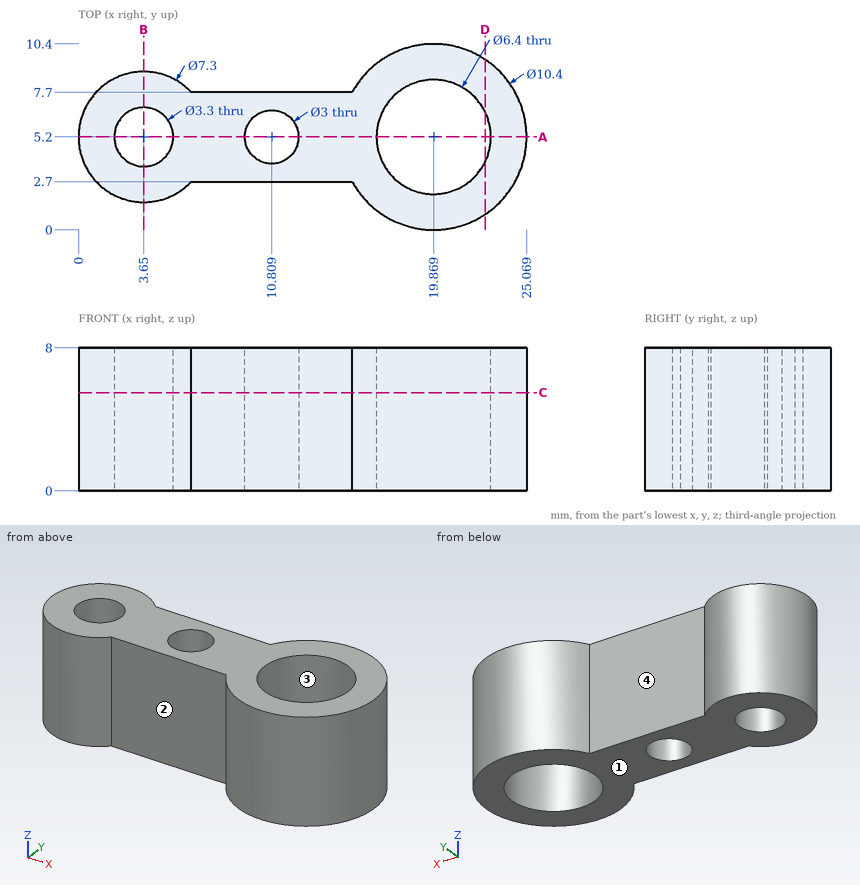
Could you check a few things on this drawing? It's one solid part, dimensions in mm from its lowest x, y, z. A direction names the side the tool comes from. Coordinates: 2 decimals unless noted, no trailing zeros. Order: outer loops, then holes, each group sorted by start corner. A loop starts at its lowest first (then second) coordinate and runs counter-clockwise, first axis right, second up. Notation, with made-up numbers: M 11,-26 L 51,-26 A24 ccw 51,-1 Z; hole C 10,-31.5 d1. An arc over 180 degrees is marked long. Use a Markdown table: item, result. Add a question column.
Q1. I want a section at D-D on x = 22.75. List the corners of the cut face in (y, z) for me.
Q2. I want a section at C-C on z = 5.5. List the corners of the cut face in (x, y) for me.
Q3. We'd pull the mould along X, two halves only. Please class the marked faces 1 and 2: pulls with the +X half, pulls with the -X half, needs draft (parallel to the pull), parting line crosses it, or undercut.
Q4. Which directions (+Z, -Z, +X, -X, +Y, -Y) give clear straight access to the entire face, cutting with the end or side of a thin tool? Please do the marked faces 3 and 4.
Q5. I'm going to push flat-ended pins straight in: pin 1 (2 mm diameter, centred on x = 18, z = 5, fed in from -Y); pin 2 (1.5 mm diameter, centred on x = 5, z = 7, fed in from -Y); pin 3 (4 mm diameter, centred on x = 14, y = 3, fed in from -Z); pin 4 (1 mm diameter, centred on x = 4.5, z = 3.5, fed in from +Y). Where does each tip first touch, or does it pass through?
Q6. I want a section at B-B on x = 3.65. List the corners of the cut face in (y, z) for me, then the cut area to 3 significant figures.
Q7. I want a section at A-A on y = 5.2. List the corners of the cut face in (x, z) for me.
Q8. If I drill on L1, parallel to X at y = 5.2, z = 6; L2, parallel to Y at x = 3.65, z = 3.5; L3, parallel to X at y = 4.5, z = 2 (1 decimal), over which ranges is the centre line in solid material (lowest first)?
Checked values:
| question | item | result |
|---|---|---|
| 1 | outline | M 0.87,0 L 3.81,0 L 3.81,8 L 0.87,8 Z; M 6.59,0 L 9.53,0 L 9.53,8 L 6.59,8 Z |
| 2 | outline | M 6.31,2.7 L 15.31,2.7 A5.2 ccw long 15.31,7.7 L 6.31,7.7 A3.65 ccw long Z; hole C 3.65,5.2 d3.3; hole C 10.81,5.2 d3; hole C 19.87,5.2 d6.4 |
| 3 | face 1 | needs draft |
| 3 | face 2 | undercut |
| 4 | face 3 | +Z, -Z |
| 4 | face 4 | +Z, -Z, +Y |
| 5 | pin 1 | y = 0.07 |
| 5 | pin 2 | y = 1.6 |
| 5 | pin 3 | z = 0 |
| 5 | pin 4 | y = 8.83 |
| 6 | outline | M 1.55,0 L 3.55,0 L 3.55,8 L 1.55,8 Z; M 6.85,0 L 8.85,0 L 8.85,8 L 6.85,8 Z |
| 6 | area | 32.0 mm² |
| 7 | outline | M 0,0 L 2,0 L 2,8 L 0,8 Z; M 5.3,0 L 9.31,0 L 9.31,8 L 5.3,8 Z; M 12.31,0 L 16.67,0 L 16.67,8 L 12.31,8 Z; M 23.07,0 L 25.07,0 L 25.07,8 L 23.07,8 Z |
| 8 | L1 | 0 to 2, 5.3 to 9.31, 12.31 to 16.67, 23.07 to 25.07 |
| 8 | L2 | 1.55 to 3.55, 6.85 to 8.85 |
| 8 | L3 | 0.1 to 2.2, 5.1 to 9.5, 12.1 to 16.7, 23 to 25 |
